Geometry: final body of the model. Coordinates: model frame, mm. A direction names the side the tool comes from. Give positions to 0.01 mm unless a question says otherwise; leave off trailing zeros. Loops run counter-clockwise (first coordinate to the right, second up) from the corner with the lowest first, then second, coordinate; pieces in that order, holes last.
from build123d import *

# Parameters (mm, degrees)
SKETCH_2_R      = 12.5
SKETCH_2_R_2    = 5
SKETCH_2_R_3    = 3
EXTRUDE_1_DEPTH = 3


with BuildPart() as part:
    # 草图2 → 凸台-拉伸1 (new body)
    # profile 1 of 4: a face of its own
    with BuildSketch(Plane(origin=(0, 0, 0), x_dir=(1, 0, 0), z_dir=(0, 1, 0))):
        with BuildLine():
            Line((7.863659035, -28.733376736), (-0.149942941, -16.843591901))
            Line((-0.149942941, -16.843591901), (4.761239815, -1.526628777))
            ThreePointArc((4.761239815, -1.526628777), (-3.515199494, -3.555752033), (-1.58113883, 4.74341649))
            Line((-1.58113883, 4.74341649), (-16.58113883, -0.25658351))
            ThreePointArc((-16.58113883, -0.25658351), (-12.076448577, -0.943789074), (-10, -5))
            ThreePointArc((-10, -5), (-16.222270381, -9.848304355), (-19.402422046, -2.629624476))
            Line((-19.402422046, -2.629624476), (-29.193931666, -20.815079176))
            ThreePointArc((-29.193931666, -20.815079176), (-15.132200589, -14.620257894), (-5.687876925, -26.741018684))
            ThreePointArc((-5.687876925, -26.741018684), (-9.34904216, -35.579853449), (-18.187876925, -39.241018684))
            Line((-18.187876925, -39.241018684), (24.980566617, -39.241018684))
            Line((24.980566617, -39.241018684), (7.863659035, -28.733376736))
        make_face()
    # profile 2 of 4: a face of its own
    with BuildSketch(Plane(origin=(0, 0, 0), x_dir=(1, 0, 0), z_dir=(0, 1, 0))):
        with Locations((-18.187876925, -26.741018684)):
            Circle(SKETCH_2_R)
    # profile 3 of 4: a face of its own
    with BuildSketch(Plane(origin=(0, 0, 0), x_dir=(1, 0, 0), z_dir=(0, 1, 0))):
        with Locations((-15, -5)):
            Circle(SKETCH_2_R_2)
        with Locations(Location((-15, -5, 0), (0, 0, 270))):
            Circle(SKETCH_2_R_3, mode=Mode.SUBTRACT)
    # profile 4 of 4: a face of its own
    with BuildSketch(Plane(origin=(0, 0, 0), x_dir=(1, 0, 0), z_dir=(0, 1, 0))):
        Circle(SKETCH_2_R_2)
        with Locations(Location((0, 0, 0), (0, 0, 270))):
            Circle(SKETCH_2_R_3, mode=Mode.SUBTRACT)
    extrude(amount=EXTRUDE_1_DEPTH)


solid = part.part
Item 1: Set-up query: faces 5 (the face through (16.54, 1.48, 34.06)), 6 (the face through (2.27, 1.48, 9.29)). Return all of +Z, -Z, +X, -X, +Y, -Y with unobstructed straight access to the full face (end or side cutting, diameter ignored); none if empty.
Values follow:
face 5: -Z, +X, +Y, -Y
face 6: +X, +Y, -Y
Item 2: Section query D-D on z = 19.5. Return loops of the section in (x, y), plus the area to 3 significant figures.
Values follow:
outline: (-28.49, 0) - (1.64, 0) - (1.64, 3) - (-28.49, 3) - close
area: 90.4 mm2
Item 3: Section query C-C on x = -15. Return loops of the section in (y, z).
Values follow:
outline: (0, -0.27) - (3, -0.27) - (3, 2) - (0, 2) - close; (0, 8) - (3, 8) - (3, 39.24) - (0, 39.24) - close
Item 4: Draft query along Z for faces 1 (the face through (0.9, 1.48, 2.86)), 2 (the face through (-8.976, 1.479, -2.278)), 3 (the face through (-9, 3, 22)), 4 (the face through (4, 1, 23)). Return one class per face: +Z half, -Z half, draft (parallel to the pull), parting line (faces both ways), or undercut.
Values follow:
face 1: undercut
face 2: -Z half
face 3: draft
face 4: undercut
Item 5: Section query B-B on z = 6.5. Return loops of the section in (x, y).
Values follow:
outline: (-21.49, 0) - (-17.6, 0) - (-17.6, 3) - (-21.49, 3) - close; (-12.4, 0) - (3.17, 0) - (3.17, 3) - (-12.4, 3) - close
Item 6: Pin query (flat end, axial travel): pin 1 (8 mm diameter, centred on x = -15, z = 5, fed in from -Y); pin 2 (1.5 mm diameter, centred on x = 13, z = 29.5, fed in from +Y). Return the tip coordinate at first contact, or that it passes through.
Values follow:
pin 1: stops at y = 0
pin 2: passes through
Item 7: Ray query, probe 1 along X at (y, z) = (1.5, 5); probe 2 along X at (y, z) = (1.4, 20); probe 3 along Z at (x, y) = (20, 2.7). Return the intervals inside material, ascending.
Values follow:
probe 1: x = -20.68 to -18, -12 to 3.65
probe 2: x = -28.76 to 1.98
probe 3: z = 36.18 to 39.24
Item 8: Section query A-A on y = 1.85. Return loops of the section in (x, z).
Values follow:
outline: (-29.19, 20.82) - (-19.4, 2.63) arc R5 ccw to (-16.58, 0.26) - (-1.58, -4.74) arc R5 ccw to (4.76, 1.53) - (-0.15, 16.84) - (7.86, 28.73) - (24.98, 39.24) - (-18.19, 39.24) arc R12.5 ccw to start; hole circle Ø6 at (-15, 5); hole circle Ø6 at (0, 0)
